Verification items for the finished model (mm, model axes). A direction names the side the tool comes from. Coordinates: 2 decimals unless noted, no trailing zeros. Order: outer loops, then holes, each group sorted by start corner. A loop starts at its lowest first (then second) coordinate and runs counter-clockwise, first axis right, second up. Notation, with made-up numbers: (-37.75, -37.5) -> (-13.75, -37.5) arc R17 ccw to (-13.75, -11.5) -> close; hole circle Ø1 at (45, 9). An arc over 180 degrees is marked (long way). Write each question's results on one line, items separated by ' | '. Start each with the question number.
(1) Cross-section at D-D on x = -0.5. Enter the section's corners in (y, z), and give its area (3 significant figures).
(2) Thickness scan on probe 1 along Y at (x, z) = (0, 1.35); probe 2 along Y at (x, z) = (1, 2.6); probe 3 along X at (y, z) = (-8.5, 1.1). Record the ranges inside material, lowest first. Write a range as [from, to].
(3) Draft check along X on faces 1 (the flat face through (16, -6.5, 1)), 2 (the flat face through (23, 0, 1)), 3 (the cylindrical face through (-11, 0, 1)). Enter one of: +X half, -X half, draft (parallel to the pull), parting line (faces both ways), or undercut.
(4) Set-up check for faces 4 (the flat face through (4.5, -21, 1.5)), 5 (the flat face through (6.5, 16, 1)), 6 (the flat face through (-16, 6.5, 1)): record each of +Z, -Z, +X, -X, +Y, -Y from which the full face is reachable in a straight line by a thin tool's end or side.
(5) Go/stop test with flat-tipped pins: pin 1 (0.9 mm diameter, centred on x = -16.5, z = 1, fed in from +Y); pin 2 (1.5 mm diameter, centred on y = 15.5, z = 1.5, fed in from +X); pin 3 (0.9 mm diameter, centred on x = 16, z = 1.5, fed in from -Y). Record where each tip stops, or that it passes through.
(6) Cross-section at C-C on z = 1.7. Give the number of separate pieces and of enclosed holes in the cut face, and give its area (3 significant figures).
(7) Cross-section at A-A on x = -17.5. Enter the section's corners in (y, z), and give its area (3 significant figures).
```python
from build123d import *

# Parameters (mm, degrees)
SKETCH1_R           = 1.5
SKETCH1_R_2         = 3.75
BOSS_EXTRUDE1_DEPTH = 3
CHAMFER1_SIZE       = 4


with BuildPart() as part:
    # Sketch1 → Boss-Extrude1 (new body)
    with BuildSketch(Plane.XY):
        with BuildLine():
            Line((-6.5, 23), (6.5, 23))
            Line((6.5, 23), (6.5, 13.518505835))
            ThreePointArc((6.5, 13.518505835), (10.606601718, 10.606601718), (13.518505835, 6.5))
            Line((13.518505835, 6.5), (23, 6.5))
            Line((23, 6.5), (23, -6.5))
            Line((23, -6.5), (13.518505835, -6.5))
            ThreePointArc((13.518505835, -6.5), (10.606601718, -10.606601718), (6.5, -13.518505835))
            Line((6.5, -13.518505835), (6.5, -23))
            Line((6.5, -23), (-6.5, -23))
            Line((-6.5, -23), (-6.5, -13.518505835))
            ThreePointArc((-6.5, -13.518505835), (-10.606601718, -10.606601718), (-13.518505835, -6.5))
            Line((-13.518505835, -6.5), (-23, -6.5))
            Line((-23, -6.5), (-23, 6.5))
            Line((-23, 6.5), (-13.518505835, 6.5))
            ThreePointArc((-13.518505835, 6.5), (-10.606601718, 10.606601718), (-6.5, 13.518505835))
            Line((-6.5, 13.518505835), (-6.5, 23))
        make_face()
        with Locations((0, 7.6)):
            Circle(SKETCH1_R, mode=Mode.SUBTRACT)
        with Locations((9.5, 0)):
            Circle(SKETCH1_R, mode=Mode.SUBTRACT)
        with Locations((-9.5, 0)):
            Circle(SKETCH1_R, mode=Mode.SUBTRACT)
        with Locations((0, -7.6)):
            Circle(SKETCH1_R, mode=Mode.SUBTRACT)
        with Locations((0, 17.5)):
            Circle(SKETCH1_R, mode=Mode.SUBTRACT)
        with Locations((17.5, 0)):
            Circle(SKETCH1_R, mode=Mode.SUBTRACT)
        with Locations((0, -17.5)):
            Circle(SKETCH1_R, mode=Mode.SUBTRACT)
        with Locations((-17.5, 0)):
            Circle(SKETCH1_R, mode=Mode.SUBTRACT)
        Circle(SKETCH1_R_2, mode=Mode.SUBTRACT)
    extrude(amount=BOSS_EXTRUDE1_DEPTH)

    # Chamfer1
    chamfer1_edges = [part.edges().sort_by_distance(p)[0] for p in [
        (23, 6.5, 1.5),
        (23, -6.5, 1.5),
        (6.5, -23, 1.5),
        (-6.5, -23, 1.5),
        (-23, -6.5, 1.5),
        (-23, 6.5, 1.5),
        (-6.5, 23, 1.5),
        (6.5, 23, 1.5),
    ]]
    chamfer(chamfer1_edges, length=CHAMFER1_SIZE)


solid = part.part
```
Results are:
1) outline: (-23, 0) -> (-18.91, 0) -> (-18.91, 3) -> (-23, 3) -> close; (-16.09, 0) -> (-9.01, 0) -> (-9.01, 3) -> (-16.09, 3) -> close; (-6.19, 0) -> (-3.72, 0) -> (-3.72, 3) -> (-6.19, 3) -> close; (3.72, 0) -> (6.19, 0) -> (6.19, 3) -> (3.72, 3) -> close; (9.01, 0) -> (16.09, 0) -> (16.09, 3) -> (9.01, 3) -> close; (18.91, 0) -> (23, 0) -> (23, 3) -> (18.91, 3) -> close | area: 81.8 mm2
2) probe 1: y = [-23, -19], [-16, -9.1], [-6.1, -3.75], [3.75, 6.1], [9.1, 16], [19, 23] | probe 2: y = [-23, -18.62], [-16.38, -8.72], [-6.48, -3.61], [3.61, 6.48], [8.72, 16.38], [18.62, 23] | probe 3: x = [-12.36, -1.2], [1.2, 12.36]
3) face 1: draft | face 2: +X half | face 3: undercut
4) face 4: +Z, -Z, +X, -Y | face 5: +Z, -Z, +X, +Y | face 6: +Z, -Z, -X, +Y
5) pin 1: stops at y = 6.5 | pin 2: stops at x = 6.5 | pin 3: stops at y = -6.5
6) separate pieces: 1 | enclosed holes: 9 | area: 983 mm2
7) outline: (-6.5, 0) -> (-1.5, 0) -> (-1.5, 3) -> (-6.5, 3) -> close; (1.5, 0) -> (6.5, 0) -> (6.5, 3) -> (1.5, 3) -> close | area: 30.0 mm2
